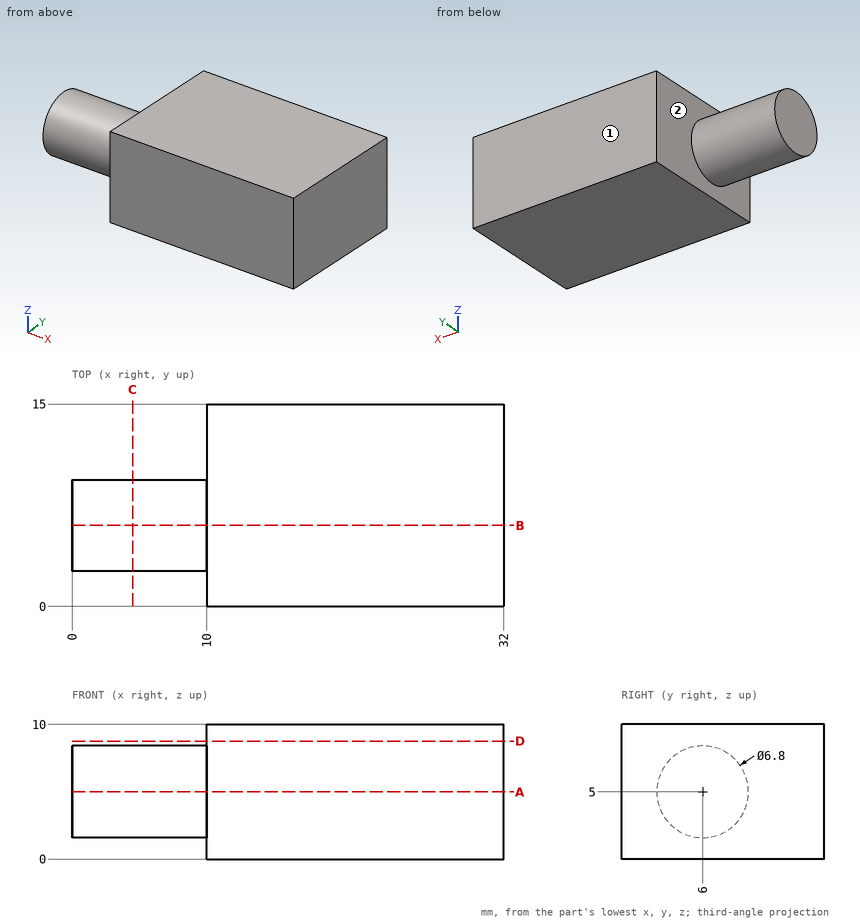
Print and shaded views of the part. All mm, measured from the part's lowest x, y and z. A direction names the side the tool comes from. Round coordinates to 2 decimals unless told otherwise and drop trailing zeros. Write each loop counter-clockwise with the first axis right and the second up, starting at its lowest first coordinate (ties: lowest second). Pieces come first, ordered by that corner, then holes.
Item 1: Probe L1, parallel to X at y = 10, z = 8.25; L2, parallel to Y at x = 5.5, z = 8; L3, parallel to Z at x = 8, y = 8.25. List the from-to ranges inside material, lowest first.
Results:
L1: x = 10 to 32
L2: y = 4.4 to 7.6
L3: z = 2.45 to 7.55
Item 2: Cut at D-D, the plane z = 8.75. Give the cut face in (x, y).
Results:
outline: (10, 0) - (32, 0) - (32, 15) - (10, 15) - close
Item 3: Cut at A-A, the plane z = 5. Give the cut face in (x, y).
Results:
outline: (0, 2.6) - (10, 2.6) - (10, 0) - (32, 0) - (32, 15) - (10, 15) - (10, 9.4) - (0, 9.4) - close
Item 4: Cut at C-C, the plane x = 4.5. Give the cut face in (y, z).
Results:
outline: circle Ø6.8 at (6, 5)
Item 5: Drop a flat-ended pin along its axis: pin 1 Ø5 at (x, z) = (4, 8.5) entering from +Y. Give the stop position or say it passes through.
Results:
pin 1: stops at y = 9.25
Item 6: Which spindle directions (+Z, -Z, +X, -X, +Y, -Y) get a long thin tool onto all of the face, cutting with end or side? Do the marked faces 1 and 2. Say none if no direction does.
Results:
face 1: +Z, -Z, +X, -X, +Y
face 2: -X
Item 7: Cut at B-B, the plane y = 6. Give the cut face in (x, z), plus the area to 3 significant figures.
Results:
outline: (0, 1.6) - (10, 1.6) - (10, 0) - (32, 0) - (32, 10) - (10, 10) - (10, 8.4) - (0, 8.4) - close
area: 288 mm2
